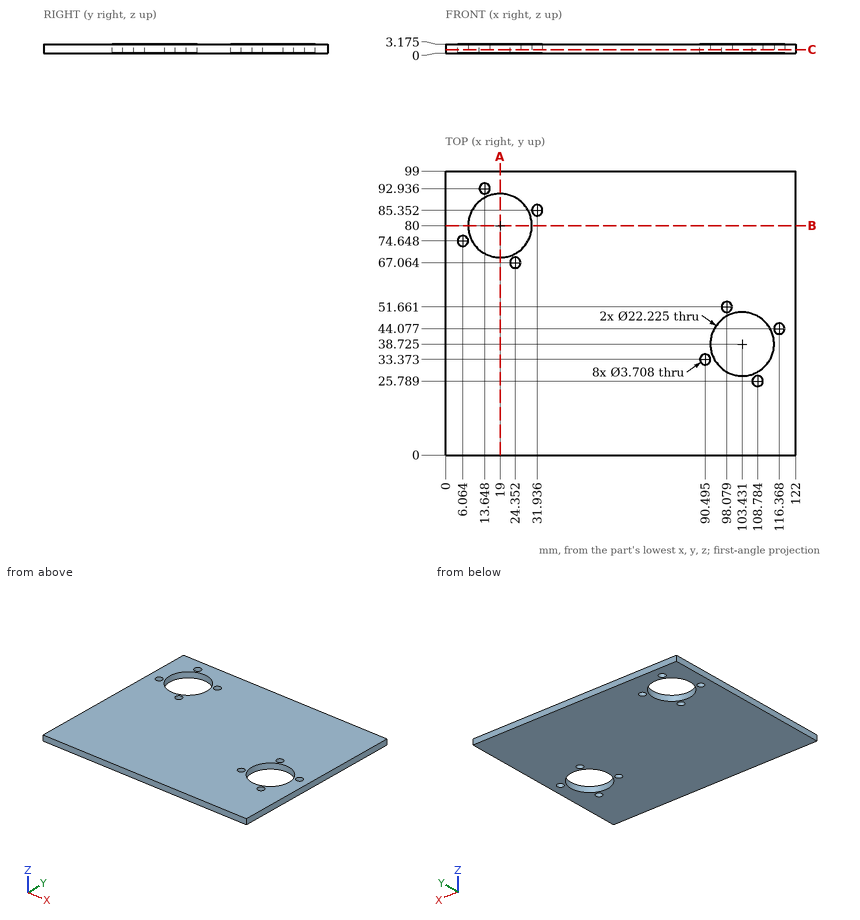
The drawing under review shows one solid part. Ordinate dimensions are in mm from its lowest x, y, z. Coordinates: 2 decimals unless noted, no trailing zeros. Loops run counter-clockwise (first coordinate to the right, second up) from the corner with the lowest first, then second, coordinate; pieces in that order, holes last. Notation, with made-up numbers: (-22, -36.5) - (-18, -36.5) arc R30 ccw to (-18, -13.5) - close; hole circle Ø10 at (-20.75, 13.25). An arc over 180 degrees is marked (long way). Return JSON: item names as keys, results as strings.
Item 1: Take a section at C-C (z = 1.25). State how many separate pieces and enclosed holes the cut face has, then the cut area to 3 significant figures.
Determined:
{"separate pieces": "1", "enclosed holes": "10", "area": "11,200 mm2"}
Item 2: Take a section at A-A (x = 19). Give the boundary of the cut face in (y, z) (1 decimal), then the cut area to 3 significant figures.
Determined:
{"outline": "(0, 0) - (68.9, 0) - (68.9, 3.2) - (0, 3.2) - close; (91.1, 0) - (99, 0) - (99, 3.2) - (91.1, 3.2) - close", "area": "244 mm2"}
Item 3: For line 1 (X direction, y = 74.5, z = 1.1) (1 decimal); line 2 (X direction, y = 85.5, z = 1.5) (1 decimal); line 3 (Y direction, x = 19, z = 1.8), list the stretches that pass through material, from the lowest coordinate up.
Determined:
{"line 1": "x = 0 to 4.2, 7.9 to 9.3, 28.7 to 122", "line 2": "x = 0 to 9.3, 28.7 to 30.1, 33.8 to 122", "line 3": "y = 0 to 68.89, 91.11 to 99"}
Item 4: Take a section at B-B (y = 80). Give the boundary of the cut face in (x, z) (1 decimal).
Determined:
{"outline": "(0, 0) - (7.9, 0) - (7.9, 3.2) - (0, 3.2) - close; (30.1, 0) - (122, 0) - (122, 3.2) - (30.1, 3.2) - close"}
Item 5: Insertion check: pin 1 (3.5 mm diameter, centred on x = 31.94, y = 85.35, fed in from +Z). The pin has a flat end and moves straight along its axis. Give the tip position at first contact, or say it passes through.
Determined:
{"pin 1": "passes through"}
